Could you check a few things on this model? Use its own coordinates, in mm. Round coordinates to 2 decimals unless told otherwise and drop trailing zeros. Write each loop counter-clockwise with the first axis right and the second up, starting at its lowest first coordinate (ties: lowest second). Pieces come first, ordered by that corner, then holes. Notation, with made-up numbers: (31.25, -20) -> (65.25, -20) arc R14 ccw to (65.25, -16) -> close; hole circle Ø3 at (87, 26). An arc over 180 degrees is marked (long way). Answer in a Markdown table with one row per item. Add a question column.
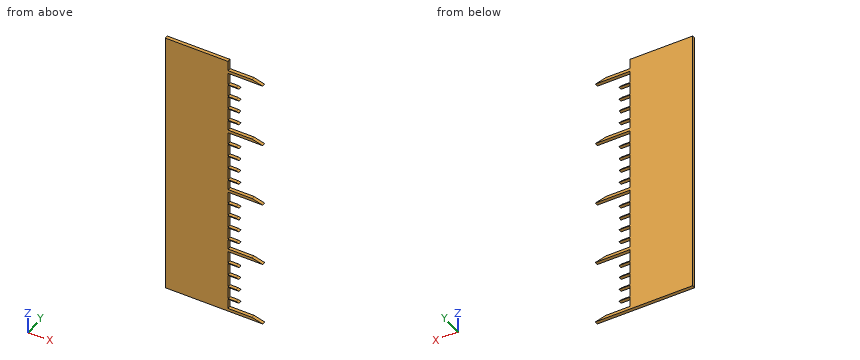
```python
from build123d import *

# Parameters (mm, degrees)
F1_DEPTH = 25


with BuildPart() as f1:
    # F0 (on Front) → F1 (new body)
    with BuildSketch(Plane.XZ):
        Polygon((0, 2100), (0, 0), (474.152878, 0), (474.152878, 5.451718), (474.152878, 22.404142), (474.152878, 100), (474.152878, 105.451718), (474.152878, 200), (474.152878, 205.451718), (474.152878, 300), (474.152878, 305.451718), (474.152878, 400), (474.152878, 405.451718), (474.152878, 500), (474.152878, 505.451718), (474.152878, 522.404142), (474.152878, 600), (474.152878, 605.451718), (474.152878, 700), (474.152878, 705.451718), (474.152878, 800), (474.152878, 805.451718), (474.152878, 900), (474.152878, 905.451718), (474.152878, 1000), (474.152878, 1005.451718), (474.152878, 1022.404142), (474.152878, 1100), (474.152878, 1105.451718), (474.152878, 1200), (474.152878, 1205.451718), (474.152878, 1300), (474.152878, 1305.451718), (474.152878, 1400), (474.152878, 1405.451718), (474.152878, 1500), (474.152878, 1505.451718), (474.152878, 1522.404142), (474.152878, 1600), (474.152878, 1605.451718), (474.152878, 1700), (474.152878, 1705.451718), (474.152878, 1800), (474.152878, 1805.451718), (474.152878, 1900), (474.152878, 1905.451718), (474.152878, 2000), (474.152878, 2022.404142), (474.152878, 2100), align=None)
        Polygon((474.152878, 5.451718), (474.152878, 0), (556.551218, 0), (535.71403, 5.451718), align=None)
        Polygon((474.152878, 22.404142), (474.152878, 5.451718), (535.71403, 5.451718), (556.551218, 0), (735.740867, 0), (655.585787, 22.404142), align=None)
        Polygon((655.585787, 2022.404142), (474.152878, 2022.404142), (474.152878, 2000), (735.740867, 2000), align=None)
        Polygon((474.152878, 105.451718), (474.152878, 100), (556.551218, 100), (535.71403, 105.451718), align=None)
        Polygon((535.71403, 1905.451718), (474.152878, 1905.451718), (474.152878, 1900), (556.551218, 1900), align=None)
        Polygon((474.152878, 205.451718), (474.152878, 200), (556.551218, 200), (535.71403, 205.451718), align=None)
        Polygon((535.71403, 1805.451718), (474.152878, 1805.451718), (474.152878, 1800), (556.551218, 1800), align=None)
        Polygon((474.152878, 305.451718), (474.152878, 300), (556.551218, 300), (535.71403, 305.451718), align=None)
        Polygon((535.71403, 1705.451718), (474.152878, 1705.451718), (474.152878, 1700), (556.551218, 1700), align=None)
        Polygon((474.152878, 405.451718), (474.152878, 400), (556.551218, 400), (535.71403, 405.451718), align=None)
        Polygon((535.71403, 1605.451718), (474.152878, 1605.451718), (474.152878, 1600), (556.551218, 1600), align=None)
        Polygon((474.152878, 505.451718), (474.152878, 500), (556.551218, 500), (535.71403, 505.451718), align=None)
        Polygon((474.152878, 522.404142), (474.152878, 505.451718), (535.71403, 505.451718), (556.551218, 500), (735.740867, 500), (655.585787, 522.404142), align=None)
        Polygon((655.585787, 1522.404142), (474.152878, 1522.404142), (474.152878, 1505.451718), (535.71403, 1505.451718), (556.551218, 1500), (735.740867, 1500), align=None)
        Polygon((535.71403, 1505.451718), (474.152878, 1505.451718), (474.152878, 1500), (556.551218, 1500), align=None)
        Polygon((474.152878, 605.451718), (474.152878, 600), (556.551218, 600), (535.71403, 605.451718), align=None)
        Polygon((535.71403, 1405.451718), (474.152878, 1405.451718), (474.152878, 1400), (556.551218, 1400), align=None)
        Polygon((474.152878, 705.451718), (474.152878, 700), (556.551218, 700), (535.71403, 705.451718), align=None)
        Polygon((535.71403, 1305.451718), (474.152878, 1305.451718), (474.152878, 1300), (556.551218, 1300), align=None)
        Polygon((474.152878, 805.451718), (474.152878, 800), (556.551218, 800), (535.71403, 805.451718), align=None)
        Polygon((535.71403, 1205.451718), (474.152878, 1205.451718), (474.152878, 1200), (556.551218, 1200), align=None)
        Polygon((474.152878, 905.451718), (474.152878, 900), (556.551218, 900), (535.71403, 905.451718), align=None)
        Polygon((535.71403, 1105.451718), (474.152878, 1105.451718), (474.152878, 1100), (556.551218, 1100), align=None)
        Polygon((474.152878, 1005.451718), (474.152878, 1000), (556.551218, 1000), (535.71403, 1005.451718), align=None)
        Polygon((474.152878, 1022.404142), (474.152878, 1005.451718), (535.71403, 1005.451718), (556.551218, 1000), (735.740867, 1000), (655.585787, 1022.404142), align=None)
    extrude(amount=F1_DEPTH)


solid = f1.part
```
(1) I need wall thicknesses on L1, parallel to Z at x = 614, y = -4; L2, parallel to X at y = -17.25, z = 1175. Which ranges of each line are inside material? Lowest first, please.
(2) For P1, Ø7.5, axis at x = 525.5, y = -10.5, coming from the -Z side; P2, Ø4, axis at x = 661.5, y = -21.5, coming from the +Z side; P3, Ø12.5, axis at x = 500.5, y = -12.5, coming from the +Z side; P4, Ø7.5, axis at y = -10.5, z = 569.5, coming from the +X side, each with a flat end and sliding along its axis, tell me the tip position at first contact or that it passes through.
(3) Suppose I cut it at B-B, the plane z = 1058. Please give me the cut outline in (x, y), then the cut area to 3 significant figures.
(4) Suppose I cut it at A-A, the plane x = 516.5. State how many separate pieces and enclosed holes the cut face has, then the cut area to 3 significant figures.
Response:
| question | item | result |
|---|---|---|
| 1 | L1 | 0 to 22.4, 500 to 522.4, 1000 to 1022.4, 1500 to 1522.4, 2000 to 2022.4 |
| 1 | L2 | 0 to 474.15 |
| 2 | P1 | z = 0 |
| 2 | P2 | z = 2021.31 |
| 2 | P3 | z = 2022.4 |
| 2 | P4 | x = 474.15 |
| 3 | outline | (0, -25) -> (474.15, -25) -> (474.15, 0) -> (0, 0) -> close |
| 3 | area | 11,900 mm² |
| 4 | separate pieces | 21 |
| 4 | enclosed holes | 0 |
| 4 | area | 4,980 mm² |
